The model under review builds one solid part; all positions refer to its coordinate system, in mm. Face numbers are marked on the shaded views. Give positions to 0.01 mm unless a question says otherwise; leave off trailing zeros. Loops run counter-clockwise (first coordinate to the right, second up) from the corner with the lowest first, then second, coordinate; pieces in that order, holes last. Notation, with made-up numbers: M 55,77 L 101,77 A11 cw 101,85 Z; hole C 80,19 d6. An arc over 180 degrees is marked long. One line per item, written item: value. Start each with the question number.
Q1. To check wall thickness, follow line 1 along Y through (x, z) = (0, 1.4); line 2 along Y through (x, z) = (-0.75, 2.45); line 3 along X through (y, z) = (21.25, 0.55). State the ranges of each line that lie inside material, in increasing order. Write a range as from..to.
Q2. We need section D-D on x = 1.25. Write out the cut boundary in (y, z), plus the area to 3 significant figures.
Q3. We need section A-A on x = 0. Write out the cut boundary in (y, z).
Q4. For pin 1 (1 mm diameter, centred on x = -0.5, y = 17, fed in from -Z), flat-tipped, find the tip position at first contact; note if it passes through.
Q5. We need section B-B on z = 0.6. Write out the cut boundary in (x, y), plus the area to 3 significant figures.
Q6. Mouldability with a two-part tool opening along X and no side actions: class the marked faces 1, 2 and 3 as released by +X, released by -X, zero draft, split by the parting line, or undercut.
Q7. We need section C-C on y = 1.75. Write out the cut boundary in (x, z).
Autodesk Inventor part; units mm, degrees
ref_plane "YZ Plane" through (0, 0, 0) normal (1, 0, 0) x (0, 1, 0)
ref_plane "XZ Plane" through (0, 0, 0) normal (0, 1, 0) x (-1, 0, 0)
ref_plane "XY Plane" through (0, 0, 0) normal (0, 0, 1) x (1, 0, 0)
sketch "Sketch1" plane through (0, 0, 0) normal (0, 0, 1) x (1, 0, 0)
  line L0 (0, 0) -> (0, 20) construction
  circle A0 centre (0, 0) radius 2.02
  circle A1 centre (0, 20) radius 1.75
  line L1 (0, 0) -> (0, 20) construction
  line L2 (4.0329, 0) -> (4.0329, 20)
  line L3 (-4.0329, 20) -> (-4.0329, 0)
  arc A2 (-4.0329, 0) -> (4.0329, 0) centre (0, 0) ccw
  arc A3 (4.0329, 20) -> (-4.0329, 20) centre (0, 20) ccw
  point P0 (0, 10)
  point P1 (0, 10)
  dimension "d0" = 20
  dimension "d2" = 4.04
  dimension "d3" = 3.5
extrude "Extrusion2" add sketch "Sketch1" along normal blind 3
properties part number "RedKangoroo_001_bar1ipt"
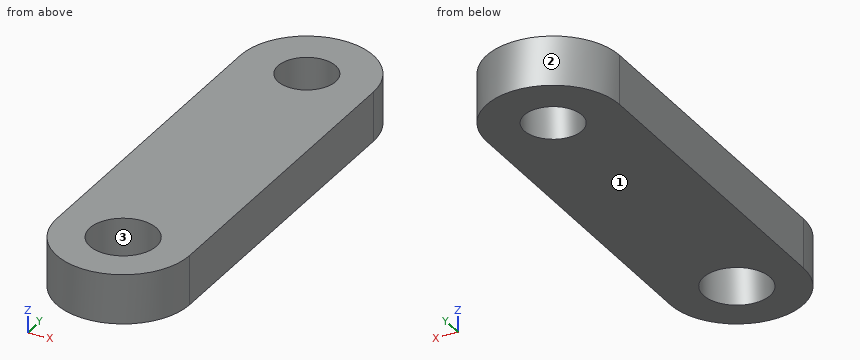
Solved:
1. line 1: -4.03..-2.02, 2.02..18.25, 21.75..24.03
1. line 2: -3.96..-1.88, 1.88..18.42, 21.58..23.96
1. line 3: -3.83..-1.22, 1.22..3.83
2. outline: M -3.83,0 L -1.59,0 L -1.59,3 L -3.83,3 Z; M 1.59,0 L 18.78,0 L 18.78,3 L 1.59,3 Z; M 21.22,0 L 23.83,0 L 23.83,3 L 21.22,3 Z
2. area: 66.1 mm2
3. outline: M -4.03,0 L -2.02,0 L -2.02,3 L -4.03,3 Z; M 2.02,0 L 18.25,0 L 18.25,3 L 2.02,3 Z; M 21.75,0 L 24.03,0 L 24.03,3 L 21.75,3 Z
4. pin 1: z = 0
5. outline: M -4.03,0 A4.03 ccw 4.03,0 L 4.03,20 A4.03 ccw -4.03,20 Z; hole C 0,0 d4.04; hole C 0,20 d3.5
5. area: 190 mm2
6. face 1: zero draft
6. face 2: split by the parting line
6. face 3: undercut
7. outline: M -4.03,0 L -1.01,0 L -1.01,3 L -4.03,3 Z; M 1.01,0 L 4.03,0 L 4.03,3 L 1.01,3 Z
